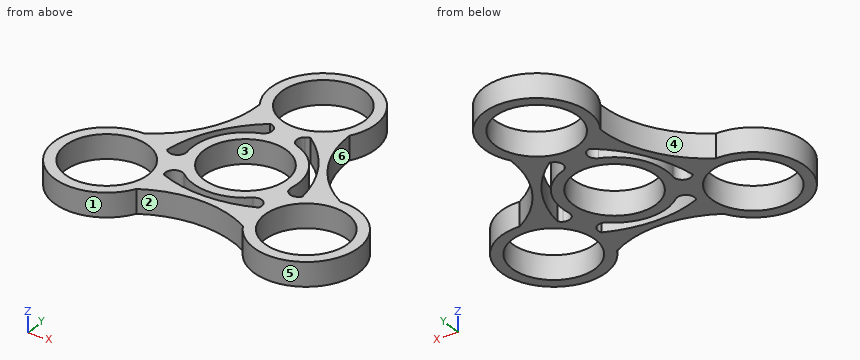
from build123d import *

# Parameters (mm, degrees)
F0_R     = 11.049
F1_DEPTH = 6.35


with BuildPart() as f1:
    # F0 (on Top) → F1 (new body)
    with BuildSketch(Plane.XY):
        with BuildLine():
            ThreePointArc((-14.078526, -21.830109), (0, -18.069067), (14.078526, -21.830109))
            ThreePointArc((14.078526, -21.830109), (38.494829, -22.225), (25.944692, -1.277306))
            ThreePointArc((25.944692, -1.277306), (15.648271, 9.034534), (11.866166, 23.107415))
            ThreePointArc((11.866166, 23.107415), (0, 44.45), (-11.866166, 23.107415))
            ThreePointArc((-11.866166, 23.107415), (-15.648271, 9.034534), (-25.944692, -1.277306))
            ThreePointArc((-25.944692, -1.277306), (-38.494829, -22.225), (-14.078526, -21.830109))
        make_face()
        with Locations((-26.396454, -15.24)):
            Circle(F0_R, mode=Mode.SUBTRACT)
        with BuildLine():
            ThreePointArc((-4.208703, 17.15905), (-3.25535, 15.05507), (-4.613117, 13.186358))
            ThreePointArc((-4.613117, 13.186358), (-12.098375, 6.985), (-13.72628, -2.598103))
            ThreePointArc((-13.72628, -2.598103), (-14.665748, -4.708319), (-16.964525, -4.934681))
            ThreePointArc((-16.964525, -4.934681), (-17.48494, -4.606139), (-17.89943, -4.1512))
            ThreePointArc((-17.89943, -4.1512), (-13.85397, 7.998594), (-5.354671, 17.576961))
            ThreePointArc((-5.354671, 17.576961), (-4.753437, 17.445472), (-4.208703, 17.15905))
        make_face(mode=Mode.SUBTRACT)
        with BuildLine():
            ThreePointArc((12.54476, -13.425761), (0, -15.997187), (-12.54476, -13.425761))
            ThreePointArc((-12.54476, -13.425761), (-12.731503, -12.839333), (-12.755821, -12.224369))
            ThreePointArc((-12.755821, -12.224369), (-11.410398, -10.346751), (-9.113163, -10.588256))
            ThreePointArc((-9.113163, -10.588256), (0, -13.97), (9.113163, -10.588256))
            ThreePointArc((9.113163, -10.588256), (11.410398, -10.346751), (12.755821, -12.224369))
            ThreePointArc((12.755821, -12.224369), (12.731503, -12.839333), (12.54476, -13.425761))
        make_face(mode=Mode.SUBTRACT)
        with Locations((26.396454, -15.24)):
            Circle(F0_R, mode=Mode.SUBTRACT)
        Circle(F0_R, mode=Mode.SUBTRACT)
        with BuildLine():
            ThreePointArc((5.354671, 17.576961), (13.85397, 7.998594), (17.89943, -4.1512))
            ThreePointArc((17.89943, -4.1512), (17.48494, -4.606139), (16.964525, -4.934681))
            ThreePointArc((16.964525, -4.934681), (14.665748, -4.708319), (13.72628, -2.598103))
            ThreePointArc((13.72628, -2.598103), (12.098375, 6.985), (4.613117, 13.186358))
            ThreePointArc((4.613117, 13.186358), (3.25535, 15.05507), (4.208703, 17.15905))
            ThreePointArc((4.208703, 17.15905), (4.753437, 17.445472), (5.354671, 17.576961))
        make_face(mode=Mode.SUBTRACT)
        with Locations((0, 30.48)):
            Circle(F0_R, mode=Mode.SUBTRACT)
    extrude(amount=F1_DEPTH)


solid = f1.part
For this review, take the finished solid that the model builds, in its own axes (mm). Face numbers are marked on the shaded views. A direction names the side the tool comes from. Round coordinates to 2 decimals unless told otherwise and drop trailing zeros. Order: outer loops, then holes, each group sorted by start corner. A loop starts at its lowest first (then second) coordinate and runs counter-clockwise, first axis right, second up. Notation, with made-up numbers: M 22.25,21 L 29.25,21 A23 cw 29.25,34 Z; hole C 44,-32.5 d5. An arc over 180 degrees is marked long. Write each question's results on one line, items separated by ' | '. Start each with the question number.
1. Add section B-B (y = 30.48). State the section outline as (x, z) points.
2. Add section C-C (y = 10). State the section outline as (x, z) points, then the cut area to 3 significant figures.
3. Add section A-A (x = 0). State the section outline as (y, z) points.
4. Draft analysis for pull direction Y (two halves, no side actions). For the marked faces 1, 2, 3 and 4, state which applies: pulls with the +Y half, pulls with the -Y half, needs draft (parallel to the pull), parting line crosses it, or undercut.
5. Tool access review of the marked faces 5 and 6: name each direction out of +Z, -Z, +X, -X, +Y, -Y from which nothing blocks a thin tool from reaching the whole face with its end or side.
6. Add section D-D (z = 5). State the section outline as (x, y) points.
7. Clearance check with flat-ended pins moving along their axes: pin 1 Ø2 at (y, z) = (4, 2) entering from +X; pin 2 Ø20 at (x, y) = (26.4, -15.24) entering from -Z; pin 3 Ø2 at (x, z) = (11, 4.5) entering from +Y; pin 4 Ø2 at (x, z) = (20, 5) entering from +Y. State where each tip first meets the part, or that it passes through.
8. To check wall thickness, follow L1, parallel to Y at x = 0.5, z = 0.75; L2, parallel to X at y = -25, z = 5.5; L3, parallel to X at y = 1, z = 0.5. State the ranges of each line that lie inside material, in increasing order. Write a range as [from, to].
Output values:
1) outline: M -13.97,0 L -11.05,0 L -11.05,6.35 L -13.97,6.35 Z; M 11.05,0 L 13.97,0 L 13.97,6.35 L 11.05,6.35 Z
2) outline: M -15.12,0 L -12.6,0 L -12.6,6.35 L -15.12,6.35 Z; M -9.76,0 L -4.7,0 L -4.7,6.35 L -9.76,6.35 Z; M 4.7,0 L 9.76,0 L 9.76,6.35 L 4.7,6.35 Z; M 12.6,0 L 15.12,0 L 15.12,6.35 L 12.6,6.35 Z | area: 96.2 mm^2
3) outline: M -18.07,0 L -16,0 L -16,6.35 L -18.07,6.35 Z; M -13.97,0 L -11.05,0 L -11.05,6.35 L -13.97,6.35 Z; M 11.05,0 L 19.43,0 L 19.43,6.35 L 11.05,6.35 Z; M 41.53,0 L 44.45,0 L 44.45,6.35 L 41.53,6.35 Z
4) face 1: parting line crosses it | face 2: pulls with the -Y half | face 3: undercut | face 4: undercut
5) face 5: +Z, -Z | face 6: +Z, -Z, +X
6) outline: M -25.94,-1.28 A13.97 ccw long -14.08,-21.83 A28.23 cw 14.08,-21.83 A13.97 ccw long 25.94,-1.28 A28.23 cw 11.87,23.11 A13.97 ccw long -11.87,23.11 A28.23 cw Z; hole C -26.4,-15.24 d22.1; hole M -17.9,-4.15 A2.3 ccw -16.96,-4.93 A2.3 ccw -13.73,-2.6 A13.97 cw -4.61,13.19 A2.3 ccw -4.21,17.16 A2.3 ccw -5.35,17.58 A31.89 ccw Z; hole M -12.76,-12.22 A2.3 ccw -12.54,-13.43 A31.89 ccw 12.54,-13.43 A2.3 ccw 12.76,-12.22 A2.3 ccw 9.11,-10.59 A13.97 cw -9.11,-10.59 A2.3 ccw Z; hole C 0,0 d22.1; hole C 0,30.48 d22.1; hole M 4.21,17.16 A2.3 ccw 4.61,13.19 A13.97 cw 13.73,-2.6 A2.3 ccw 16.96,-4.93 A2.3 ccw 17.9,-4.15 A31.89 ccw 5.35,17.58 A2.3 ccw Z; hole C 26.4,-15.24 d22.1
7) pin 1: x = 20.32 | pin 2: through | pin 3: y = 40.24 | pin 4: y = 4.39
8) L1: [-18.07, -15.99], [-13.96, -11.04], [11.04, 19.44], [41.52, 44.44] | L2: [-36.39, -31.58], [-21.22, -16.4], [16.4, 21.22], [31.58, 36.39] | L3: [-22.59, -16.85], [-13.93, -11], [11, 13.93], [16.85, 22.59]
